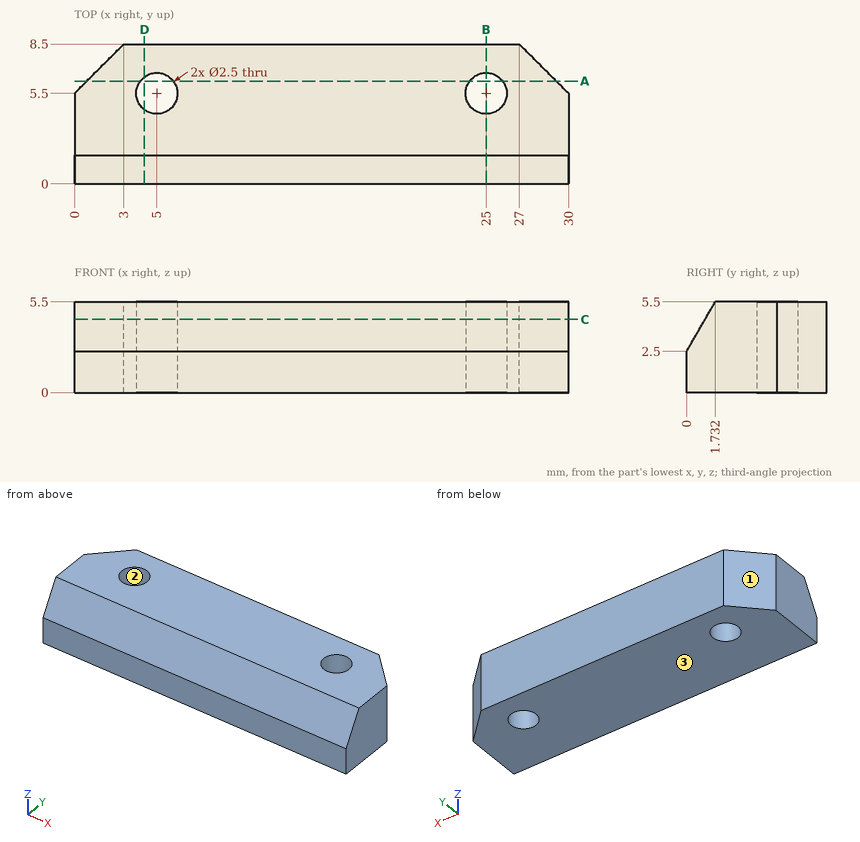
Can you work these out from the drawing? Everything is in mm from the part's minimum corner. Coordinates: 2 decimals unless noted, no trailing zeros. Order: outer loops, then holes, each group sorted by start corner. A loop starts at its lowest first (then second) coordinate and runs counter-clockwise, first axis right, second up. Notation, with made-up numbers: M -7,79.25 L 48,79.25 A22 ccw 48,90.25 Z; hole C 84.5,-24.5 d3. An arc over 180 degrees is marked long. Answer as CSV lines item,"result". Start each with the question number.
1. I want a section at C-C, the plane z = 4.45. Write out the boundary of the cut face in (x, y).
2. I want a section at D-D, the plane x = 4.25. Write out the boundary of the cut face in (y, z).
3. I want a section at A-A, the plane y = 6.25. Write out the boundary of the cut face in (x, z), and give its area (3 significant figures).
4. We'd pull the mould along X, two halves only. Please class the marked faces 1, 2 and 3: released by +X, released by -X, zero draft, split by the parting line, or undercut.
5. I need wall thicknesses on line 1 (Y direction, x = 25, z = 1.75); line 2 (Y direction, x = 28.75, z = 1.1); line 3 (X direction, y = 4.75, z = 3.5). Which ranges of each line are inside material? Lowest first, please. Write a range as [from, to].
6. I want a section at B-B, the plane x = 25. Write out the boundary of the cut face in (y, z), and give its area (3 significant figures).
7. For pin 1 (4 mm diameter, centred on x = 17, y = 4.5, fed in from -Z), with a flat end and sliding along its axis, tell me the tip position at first contact or that it passes through.
Recorded:
1,outline,"M 0,1.13 L 30,1.13 L 30,5.5 L 27,8.5 L 3,8.5 L 0,5.5 Z; hole C 5,5.5 d2.5; hole C 25,5.5 d2.5"
2,outline,"M 0,0 L 4.5,0 L 4.5,5.5 L 1.73,5.5 L 0,2.5 Z; M 6.5,0 L 8.5,0 L 8.5,5.5 L 6.5,5.5 Z"
3,outline,"M 0.75,0 L 4,0 L 4,5.5 L 0.75,5.5 Z; M 6,0 L 24,0 L 24,5.5 L 6,5.5 Z; M 26,0 L 29.25,0 L 29.25,5.5 L 26,5.5 Z"
3,area,"135 mm2"
4,face 1,"released by -X"
4,face 2,"undercut"
4,face 3,"zero draft"
5,line 1,"y = [0, 4.25], [6.75, 8.5]"
5,line 2,"y = [0, 6.75]"
5,line 3,"x = [0, 4], [6, 24], [26, 30]"
6,outline,"M 0,0 L 4.25,0 L 4.25,5.5 L 1.73,5.5 L 0,2.5 Z; M 6.75,0 L 8.5,0 L 8.5,5.5 L 6.75,5.5 Z"
6,area,"30.4 mm2"
7,pin 1,"stops at z = 0"
